```python
from build123d import *

# Parameters (mm, degrees)
SKETCH2_W           = 53
SKETCH2_H           = 43
BOSS_EXTRUDE1_DEPTH = 10
SKETCH3_W           = 38.2
SKETCH3_H           = 8.2
BOSS_EXTRUDE2_DEPTH = 8
SKETCH4_W           = 24
SKETCH4_H           = 8.2
CUT_EXTRUDE1_DEPTH  = 3
SKETCH5_R           = 1.5
CUT_EXTRUDE2_DEPTH  = 69.740381145
SKETCH6_W           = 53
SKETCH6_H           = 6
BOSS_EXTRUDE4_DEPTH = 8
SKETCH7_R           = 1.75
CUT_EXTRUDE3_DEPTH  = 76.723180071
SKETCH8_W           = 43
SKETCH8_H           = 17
CUT_EXTRUDE4_DEPTH  = 4


with BuildPart() as part:
    # Sketch2 → Boss-Extrude1 (new body)
    with BuildSketch(Plane(origin=(0, 0, 0), x_dir=(1, 0, 0), z_dir=(0, 1, 0))):
        with Locations((26.5, 21.5)):
            Rectangle(SKETCH2_W, SKETCH2_H)
    extrude(amount=BOSS_EXTRUDE1_DEPTH)

    # Sketch3 → Boss-Extrude2 (add)
    with BuildSketch(Plane.XY):
        with Locations((25.59901915, 4.1)):
            Rectangle(SKETCH3_W, SKETCH3_H)
    extrude(amount=BOSS_EXTRUDE2_DEPTH)

    # Sketch4 → Cut-Extrude1 (cut)
    with BuildSketch(Plane.XY.offset(8)):
        with Locations((25.49901915, 4.1)):
            Rectangle(SKETCH4_W, SKETCH4_H)
    extrude(amount=-CUT_EXTRUDE1_DEPTH, mode=Mode.SUBTRACT)

    # Sketch5 → Cut-Extrude2 (cut, through all)
    with BuildSketch(Plane(origin=(0, 8.2, 0), x_dir=(1, 0, 0), z_dir=(0, 1, 0))):
        with Locations(Location((40.49901915, -4.5, 0), (0, 0, 270))):
            Circle(SKETCH5_R)
        with Locations(Location((10.49901915, -4.5, 0), (0, 0, 270))):
            Circle(SKETCH5_R)
    extrude(amount=-CUT_EXTRUDE2_DEPTH, mode=Mode.SUBTRACT)

    # Sketch6 → Boss-Extrude4 (add)
    with BuildSketch(Plane(origin=(0, 10, 0), x_dir=(1, 0, 0), z_dir=(0, 1, 0))):
        with Locations((26.5, 40)):
            Rectangle(SKETCH6_W, SKETCH6_H)
    extrude(amount=BOSS_EXTRUDE4_DEPTH)

    # Sketch7 → Cut-Extrude3 (cut, through all)
    with BuildSketch(Plane(origin=(0, 0, -43), x_dir=(-1, 0, 0), z_dir=(0, 0, -1))):
        with Locations((-41.25, 12)):
            Circle(SKETCH7_R)
        with Locations((-26.25, 12)):
            Circle(SKETCH7_R)
        with Locations((-11.25, 12)):
            Circle(SKETCH7_R)
    extrude(amount=-CUT_EXTRUDE3_DEPTH, mode=Mode.SUBTRACT)

    # Sketch8 → Cut-Extrude4 (cut)
    with BuildSketch(Plane(origin=(0, 10, 0), x_dir=(1, 0, 0), z_dir=(0, 1, 0))):
        with Locations((26.5, 28.5)):
            Rectangle(SKETCH8_W, SKETCH8_H)
    extrude(amount=-CUT_EXTRUDE4_DEPTH, mode=Mode.SUBTRACT)


solid = part.part
```
CAD build for the part. Positions are in the model's coordinates, mm. A direction names the side the tool comes from. Give positions to 0.01 mm unless a question says otherwise; leave off trailing zeros. Order: outer loops, then holes, each group sorted by start corner. A loop starts at its lowest first (then second) coordinate and runs counter-clockwise, first axis right, second up.
(1) Saw through at D-D, the plane y = 5.25. Give the cut face in (x, z).
(2) Saw through at A-A, the plane x = 26.25. Give the cut face in (y, z), then the cut area to 3 significant figures.
(3) Saw through at C-C, the plane z = -35.5. Give the cut face in (x, y).
(4) Mould opens along Z. For faces 5 (the flat face through (26, 6, -29)), 6 (the flat face through (26, 0, -18)), 7 (the flat face through (10, 4, 8)) say: released by +Z, released by -Z, zero draft, split by the parting line, or undercut.
(5) Flat gauge pins, fed straight in: pin 1 (4.5 mm diameter, centred on x = 11.25, y = 12, fed in from +Z); pin 2 (10 mm diameter, centred on x = 30, z = -23.5, fed in from +Y); pin 3 (6 mm diameter, centred on x = 26.5, z = -28, fed in from +Y). Where does each tip first touch, or does it go through?
(6) Drill centre lines: L1, parallel to X at y = 5.25, z = 4.5; L2, parallel to X at y = 8.75, z = -21.5; L3, parallel to Y at x = 26.25, z = -40.25. Where is each one in solid material? Low to high.
(7) Saw through at B-B, the plane y = 12. Give the cut face in (x, z), then the cut area to 3 significant figures.
(8) Tool access for faces 1 (the flat face through (5, 8, -28)), 2 (the flat face through (44.699, 4, 4)), 3 (the flat face through (13.499, 4, 7)), 4 (the flat face through (6.499, 4, 4)): list every direction of +Z, -Z, +X, -X, +Y, -Y with a clear straight run to the whole face (end or side of a thin tool).
Results found:
1. outline: (0, -43) - (53, -43) - (53, 0) - (44.7, 0) - (44.7, 8) - (37.5, 8) - (37.5, 5) - (13.5, 5) - (13.5, 8) - (6.5, 8) - (6.5, 0) - (0, 0) - close; hole circle Ø3 at (10.5, 4.5); hole circle Ø3 at (40.5, 4.5)
2. outline: (0, -43) - (10.25, -43) - (10.25, -37) - (6, -37) - (6, -20) - (10, -20) - (10, 0) - (8.2, 0) - (8.2, 5) - (0, 5) - close; (13.75, -43) - (18, -43) - (18, -37) - (13.75, -37) - close
2. area: 430 mm2
3. outline: (0, 0) - (53, 0) - (53, 10) - (48, 10) - (48, 6) - (5, 6) - (5, 10) - (0, 10) - close
4. face 5: undercut
4. face 6: zero draft
4. face 7: released by +Z
5. pin 1: stops at z = 0
5. pin 2: stops at y = 10
5. pin 3: stops at y = 6
6. L1: x = 6.5 to 9, 12 to 39, 42 to 44.7
6. L2: x = 0 to 5, 48 to 53
6. L3: y = 0 to 10.25, 13.75 to 18
7. outline: (0, -43) - (9.5, -43) - (9.5, -37) - (0, -37) - close; (13, -43) - (24.5, -43) - (24.5, -37) - (13, -37) - close; (28, -43) - (39.5, -43) - (39.5, -37) - (28, -37) - close; (43, -43) - (53, -43) - (53, -37) - (43, -37) - close
7. area: 255 mm2
8. face 1: +Y
8. face 2: +Z, +X, +Y, -Y
8. face 3: +Z, +Y, -Y
8. face 4: +Z, -X, +Y, -Y
